Drawing for the job (mm, zero at the part's lowest x, y, z). A direction names the side the tool comes from. Give positions to 0.01 mm unless a question says otherwise; leave off trailing zeros. Order: outer loops, then holes, each group sorted by start corner. A loop starts at its lowest first (then second) coordinate and runs counter-clockwise, first axis right, second up. Notation, with made-up numbers: (2.25, 56.5) -> (45.25, 56.5) arc R22 ccw to (45.25, 71.5) -> close; hole circle Ø2 at (59, 80). An arc over 180 degrees is marked (long way). Use a Markdown table: item, result. Add a question column.
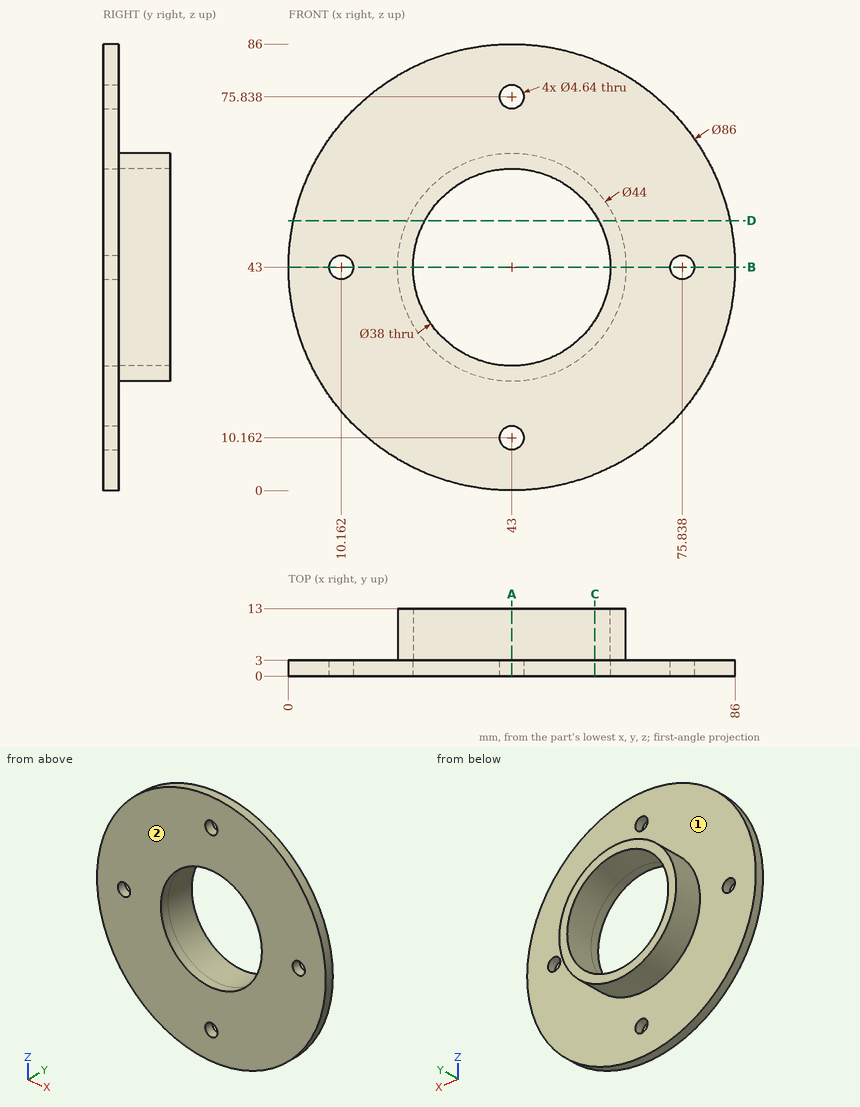
(1) Band-saw the part on A-A on x = 43. Give the cut face in (y, z).
(2) Band-saw the part on B-B on z = 43. Give the cut face in (x, y), plus the area to 3 significant figures.
(3) Tool access for the marked faces 1 and 2: list every direction of +Z, -Z, +X, -X, +Y, -Y with a clear straight run to the whole face (end or side of a thin tool).
(4) Band-saw the part on C-C on x = 59. Give the cut face in (y, z), plus the area to 3 significant figures.
(5) Wall check: probe 1 along Z at (x, y) = (43, 2.2); probe 2 along Z at (x, y) = (43, 9.5). Give the ranges that are in metal, low to high.
(6) Band-saw the part on D-D on z = 52. Give the cut face in (x, y) (1 decimal), plus the area to 3 significant figures.
(7) Pin check, flat tips, straight feed: pin 1 Ø3 at (y, z) = (3.5, 22.5) entering from -X; pin 2 Ø6 at (x, z) = (10.16, 43) entering from +Y; pin 3 Ø1.5 at (y, z) = (9.5, 63.5) entering from +X; pin 4 Ø7.5 at (x, z) = (43, 75.84) entering from -Y. Stop position of each tip, or through.
Response:
| question | item | result |
|---|---|---|
| 1 | outline | (0, 0) -> (3, 0) -> (3, 7.84) -> (0, 7.84) -> close; (0, 12.48) -> (3, 12.48) -> (3, 21) -> (13, 21) -> (13, 24) -> (0, 24) -> close; (0, 62) -> (13, 62) -> (13, 65) -> (3, 65) -> (3, 73.52) -> (0, 73.52) -> close; (0, 78.16) -> (3, 78.16) -> (3, 86) -> (0, 86) -> close |
| 2 | outline | (0, 0) -> (7.84, 0) -> (7.84, 3) -> (0, 3) -> close; (12.48, 0) -> (24, 0) -> (24, 13) -> (21, 13) -> (21, 3) -> (12.48, 3) -> close; (62, 0) -> (73.52, 0) -> (73.52, 3) -> (65, 3) -> (65, 13) -> (62, 13) -> close; (78.16, 0) -> (86, 0) -> (86, 3) -> (78.16, 3) -> close |
| 2 | area | 176 mm² |
| 3 | face 1 | +Y |
| 3 | face 2 | +Z, -Z, +X, -X, -Y |
| 4 | outline | (0, 3.09) -> (3, 3.09) -> (3, 27.9) -> (13, 27.9) -> (13, 32.75) -> (0, 32.75) -> close; (0, 53.25) -> (13, 53.25) -> (13, 58.1) -> (3, 58.1) -> (3, 82.91) -> (0, 82.91) -> close |
| 4 | area | 275 mm² |
| 5 | probe 1 | z = 0 to 7.84, 12.48 to 24, 62 to 73.52, 78.16 to 86 |
| 5 | probe 2 | z = 21 to 24, 62 to 65 |
| 6 | outline | (1, 0) -> (26.3, 0) -> (26.3, 13) -> (22.9, 13) -> (22.9, 3) -> (1, 3) -> close; (59.7, 0) -> (85, 0) -> (85, 3) -> (63.1, 3) -> (63.1, 13) -> (59.7, 13) -> close |
| 6 | area | 219 mm² |
| 7 | pin 1 | stops at x = 4.47 |
| 7 | pin 2 | stops at y = 3 |
| 7 | pin 3 | stops at x = 52.69 |
| 7 | pin 4 | stops at y = 0 |
